The model under review builds one solid part; all positions refer to its coordinate system, in mm. Face numbers are marked on the shaded views. A direction names the side the tool comes from. Round coordinates to 2 decimals unless told otherwise and drop trailing zeros. Loops run counter-clockwise (first coordinate to the right, second up) from the corner with the lowest first, then second, coordinate; pieces in that order, holes last. Notation, with made-up numbers: (34.25, -2.5) -> (91.25, -2.5) arc R10 ccw to (91.25, 12.5) -> close; hole circle Ø11 at (36.25, 41). An arc over 180 degrees is marked (long way). Return JSON: item names as keys, results as strings. Group by question number.
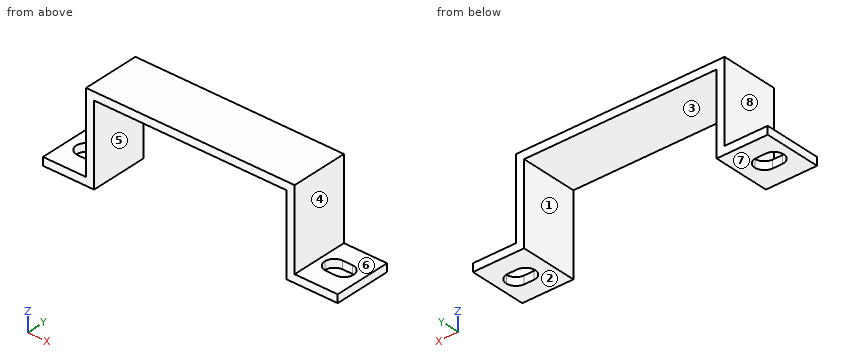
```python
from build123d import *

# Parameters (mm, degrees)
F0_W     = 6.725
F0_H     = 1.25
F0_W_2   = 1.25
F1_DEPTH = 8.95
F3_DEPTH = 25


with BuildPart() as f1:
    # F0 (on Front) → F1 (new body)
    with BuildSketch(Plane.XZ):
        with Locations((-19.6375, 0.625)):
            Rectangle(F0_W, F0_H)
        with Locations((-15.65, 0.625)):
            Rectangle(F0_W_2, F0_H)
        Polygon((-16.275, 13.8), (-16.275, 1.25), (-15.025, 1.25), (-15.025, 12.55), (15.025, 12.55), (15.025, 1.25), (16.275, 1.25), (16.275, 13.8), align=None)
        with Locations((15.65, 0.625)):
            Rectangle(F0_W_2, F0_H)
        with Locations((19.6375, 0.625)):
            Rectangle(F0_W, F0_H)
    extrude(amount=F1_DEPTH)

    # F2 (on face) → F3 (cut)
    with BuildSketch(Plane.XY.offset(1.25)):
        with BuildLine():
            ThreePointArc((-19.39, -3.1759618943), (-19.0282285677, -3.0261112606), (-18.64, -2.975))
            Line((-18.64, -2.975), (-20.14, -2.975))
            ThreePointArc((-20.14, -2.975), (-19.7517714323, -3.0261112606), (-19.39, -3.1759618943))
        make_face()
        with BuildLine():
            ThreePointArc((-19.39, -5.7740381057), (-20.14, -4.475), (-19.39, -3.1759618943))
            ThreePointArc((-19.39, -3.1759618943), (-19.7517714323, -3.0261112606), (-20.14, -2.975))
            ThreePointArc((-20.14, -2.975), (-21.64, -4.475), (-20.14, -5.975))
            ThreePointArc((-20.14, -5.975), (-19.7517714323, -5.9238887394), (-19.39, -5.7740381057))
        make_face()
        with BuildLine():
            ThreePointArc((-19.39, -5.7740381057), (-18.8409618943, -5.225), (-18.64, -4.475))
            ThreePointArc((-18.64, -4.475), (-18.8409618943, -3.725), (-19.39, -3.1759618943))
            ThreePointArc((-19.39, -3.1759618943), (-20.14, -4.475), (-19.39, -5.7740381057))
        make_face()
        with BuildLine():
            Line((-18.64, -4.475), (-17.14, -4.475))
            ThreePointArc((-17.14, -4.475), (-17.5793398282, -3.4143398282), (-18.64, -2.975))
            ThreePointArc((-18.64, -2.975), (-19.0282285677, -3.0261112606), (-19.39, -3.1759618943))
            ThreePointArc((-19.39, -3.1759618943), (-18.8409618943, -3.725), (-18.64, -4.475))
        make_face()
        with BuildLine():
            ThreePointArc((-18.64, -5.975), (-17.5793398282, -5.5356601718), (-17.14, -4.475))
            Line((-17.14, -4.475), (-18.64, -4.475))
            ThreePointArc((-18.64, -4.475), (-18.8409618943, -5.225), (-19.39, -5.7740381057))
            ThreePointArc((-19.39, -5.7740381057), (-19.0282285677, -5.9238887394), (-18.64, -5.975))
        make_face()
        with BuildLine():
            Line((-20.14, -5.975), (-18.64, -5.975))
            ThreePointArc((-18.64, -5.975), (-19.0282285677, -5.9238887394), (-19.39, -5.7740381057))
            ThreePointArc((-19.39, -5.7740381057), (-19.7517714323, -5.9238887394), (-20.14, -5.975))
        make_face()
        with BuildLine():
            Line((20.14, -2.975), (18.64, -2.975))
            ThreePointArc((18.64, -2.975), (19.0282285677, -3.0261112606), (19.39, -3.1759618943))
            ThreePointArc((19.39, -3.1759618943), (19.7517714323, -3.0261112606), (20.14, -2.975))
        make_face()
        with BuildLine():
            ThreePointArc((18.64, -2.975), (17.5793398282, -3.4143398282), (17.14, -4.475))
            Line((17.14, -4.475), (18.64, -4.475))
            ThreePointArc((18.64, -4.475), (18.8409618943, -3.725), (19.39, -3.1759618943))
            ThreePointArc((19.39, -3.1759618943), (19.0282285677, -3.0261112606), (18.64, -2.975))
        make_face()
        with BuildLine():
            ThreePointArc((19.39, -3.1759618943), (18.8409618943, -3.725), (18.64, -4.475))
            ThreePointArc((18.64, -4.475), (18.8409618943, -5.225), (19.39, -5.7740381057))
            ThreePointArc((19.39, -5.7740381057), (19.9390381057, -5.225), (20.14, -4.475))
            ThreePointArc((20.14, -4.475), (19.9390381057, -3.725), (19.39, -3.1759618943))
        make_face()
        with BuildLine():
            ThreePointArc((20.14, -2.975), (19.7517714323, -3.0261112606), (19.39, -3.1759618943))
            ThreePointArc((19.39, -3.1759618943), (19.9390381057, -3.725), (20.14, -4.475))
            ThreePointArc((20.14, -4.475), (19.9390381057, -5.225), (19.39, -5.7740381057))
            ThreePointArc((19.39, -5.7740381057), (19.7517714323, -5.9238887394), (20.14, -5.975))
            ThreePointArc((20.14, -5.975), (21.2006601718, -5.5356601718), (21.64, -4.475))
            ThreePointArc((21.64, -4.475), (21.2006601718, -3.4143398282), (20.14, -2.975))
        make_face()
        with BuildLine():
            ThreePointArc((19.39, -5.7740381057), (19.0282285677, -5.9238887394), (18.64, -5.975))
            Line((18.64, -5.975), (20.14, -5.975))
            ThreePointArc((20.14, -5.975), (19.7517714323, -5.9238887394), (19.39, -5.7740381057))
        make_face()
        with BuildLine():
            Line((18.64, -4.475), (17.14, -4.475))
            ThreePointArc((17.14, -4.475), (17.5793398282, -5.5356601718), (18.64, -5.975))
            ThreePointArc((18.64, -5.975), (19.0282285677, -5.9238887394), (19.39, -5.7740381057))
            ThreePointArc((19.39, -5.7740381057), (18.8409618943, -5.225), (18.64, -4.475))
        make_face()
    extrude(amount=-F3_DEPTH, mode=Mode.SUBTRACT)


solid = f1.part
```
1. Draft analysis for pull direction X (two halves, no side actions). For the marked faces 1, 2, 3 and 4, state which applies: pulls with the +X half, pulls with the -X half, needs draft (parallel to the pull), parting line crosses it, or undercut.
2. For P1, Ø2.5, axis at y = -5, z = 9, coming from the -X side (3 decimals); P2, Ø2, axis at y = -4, z = 9, coming from the +X side (3 decimals); P3, Ø3.5, axis at x = -19.5, y = -3.5, coming from the +Z side, all flat-tipped, find the tip position at first contact; note any pin that passes through.
3. Tool access review of the marked faces 5, 6, 7 and 8: name each direction out of +Z, -Z, +X, -X, +Y, -Y from which nothing blocks a thin tool from reaching the whole face with its end or side.
4. Wall thickness on line 1 (X direction, y = -6, z = 10.25) (3 decimals); line 2 (Z direction, x = 6.5, y = -2.75); line 3 (Z direction, x = -18.5, y = -1.5): over which ranges is each line inside the solid? List them lowest first.
5. We need section B-B, the plane y = -7. Write out the cut boundary in (x, z) (3 decimals).
6. We need section A-A, the plane z = 7.75. Write out the cut boundary in (x, y) (3 decimals).
Check sheet entries:
{
 "1": {"face 1": "undercut", "face 2": "needs draft", "face 3": "undercut", "face 4": "pulls with the +X half"},
 "2": {"P1": "stops at x = -16.275", "P2": "stops at x = 16.275", "P3": "stops at z = 1.25"},
 "3": {"face 5": "-Z, +Y, -Y", "face 6": "+Z, +X, +Y, -Y", "face 7": "-Z, +X, -X, +Y, -Y", "face 8": "+Z, -X, +Y, -Y"},
 "4": {"line 1": "x = -16.275 to -15.025, 15.025 to 16.275", "line 2": "z = 12.55 to 13.8", "line 3": "z = 0 to 1.25"},
 "5": {"outline": "(-23, 0) -> (-15.025, 0) -> (-15.025, 12.55) -> (15.025, 12.55) -> (15.025, 0) -> (23, 0) -> (23, 1.25) -> (16.275, 1.25) -> (16.275, 13.8) -> (-16.275, 13.8) -> (-16.275, 1.25) -> (-23, 1.25) -> close"},
 "6": {"outline": "(-16.275, -8.95) -> (-15.025, -8.95) -> (-15.025, 0) -> (-16.275, 0) -> close; (15.025, -8.95) -> (16.275, -8.95) -> (16.275, 0) -> (15.025, 0) -> close"}
}
